Work out the finished part from the listing and answer in its coordinate system (mm). Face numbers are marked on the shaded views. A direction names the side the tool comes from. Coordinates: 2 decimals unless noted, no trailing zeros. Order: outer loops, then holes, each group sorted by start corner. A loop starts at its lowest first (then second) coordinate and runs counter-clockwise, first axis right, second up. Notation, with made-up numbers: M 4,-40 L 8,-40 A33 ccw 8,-3 Z; hole C -26.5,44 d2. An arc over 180 degrees is marked long. Use a Markdown table: item, result. Add a question column.
from build123d import *

# Parameters (mm, degrees)
SKETCH016_R           = 9.016071
PAD004_DEPTH          = 2
REVOLUTION003_ANGLE   = -140
POLARPATTERN001_COUNT = 2


with BuildPart() as part:
    # Sketch016 → Pad004 (new body)
    with BuildSketch(Plane.XY):
        Circle(SKETCH016_R)
    extrude(amount=-PAD004_DEPTH)

    # Sketch018 → Revolution003 (revolve)
    with BuildSketch(Plane.YZ):
        with BuildLine():
            Line((1.8, 0), (1.8, 8))
            Line((1.8, 8), (6.25, 8))
            ThreePointArc((6.25, 6), (6.5, 7), (6.25, 8))
            Line((6.25, 6), (6.25, 0))
            Line((6.25, 0), (1.8, 0))
        make_face()
    revolution003 = revolve(axis=Axis((0, 0, 0), (0, 0, 1)), revolution_arc=REVOLUTION003_ANGLE)

    # PolarPattern001: Revolution003 ×2 about axis
    polarpattern001_axis = Axis((0, 0, 0), (0, 0, 1))
    for i in range(1, POLARPATTERN001_COUNT):
        add(revolution003.rotate(polarpattern001_axis, i * 360 / POLARPATTERN001_COUNT))


solid = part.part
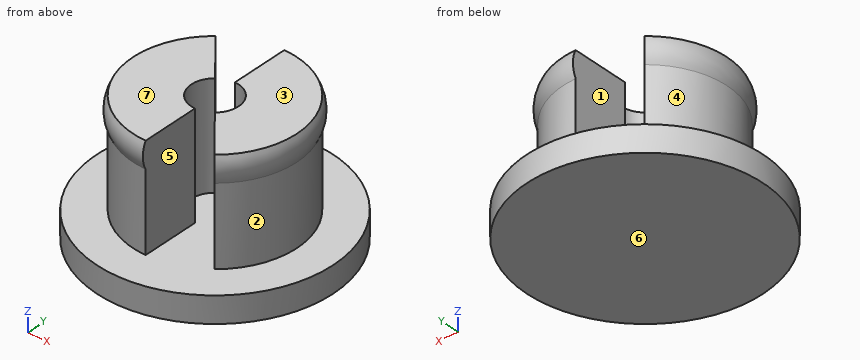
(1) Given P1, Ø1, axis at y = 5, z = 6, coming from the -X side; P2, Ø5, axis at x = 4, z = 4.5, coming from the -Y side; P3, Ø6, axis at x = 2.5, z = 6, coming from the +Y side, each flat-ended and moving along its own axis, determine where each tip first touches the part or whether it passes through.
(2) Which of the six approach directions +Z, -Z, +X, -X, +Y, -Y give full straight-line access (tool end or side, diameter ignored) to the marked faces 4, 5, 6 and 7?
(3) The mould has two halves that part along Z. Classify the marked faces 1, 2 and 3: pulls with the +Z half, pulls with the -Z half, needs draft (parallel to the pull), parting line crosses it, or undercut.
(4) Straight lines are drawn through the part: line 1 (Z direction, x = 1.5, y = -0.25); line 2 (X direction, y = 2.5, z = 2); line 3 (X direction, y = 0.25, z = 4) (3 decimals). For each, find the intervals that lie inside material, in ascending order.
(5) A cutting plane is placed at B-B on z = 1. Write down the section's boundary in (x, y), plus the area to 3 significant figures.
(6) A cutting plane is placed at C-C on x = 8. Write down the section's boundary in (y, z), plus the area to 3 significant figures.
(7) A cutting plane is placed at A-A on y = 0. Write down the section's boundary in (x, z) (3 decimals).
From the geometry:
| question | item | result |
|---|---|---|
| 1 | P1 | stops at x = -4.43 |
| 1 | P2 | stops at y = -4.98 |
| 1 | P3 | stops at y = 6.5 |
| 2 | face 4 | -X |
| 2 | face 5 | +Z, -Y |
| 2 | face 6 | -Z, +X, -X, +Y, -Y |
| 2 | face 7 | +Z, +X, -X, +Y, -Y |
| 3 | face 1 | needs draft |
| 3 | face 2 | undercut |
| 3 | face 3 | pulls with the +Z half |
| 4 | line 1 | z = -2 to 0 |
| 4 | line 2 | x = -5.73 to -2.1, 0 to 5.73 |
| 4 | line 3 | x = -6.245 to -1.783, 1.783 to 6.245 |
| 5 | outline | M -4.02,4.79 A6.25 ccw 0,-6.25 L 0,-1.8 A1.8 cw -1.16,1.38 Z; M 0,1.8 A1.8 cw 1.16,-1.38 L 4.02,-4.79 A6.25 ccw 0,6.25 Z |
| 5 | area | 87.5 mm2 |
| 6 | outline | M -4.16,-2 L 4.16,-2 L 4.16,0 L -4.16,0 Z |
| 6 | area | 16.6 mm2 |
| 7 | outline | M -9.016,-2 L 9.016,-2 L 9.016,0 L 6.25,0 L 6.25,6 A2.125 ccw 6.25,8 L 1.8,8 L 1.8,0 L -1.8,0 L -1.8,8 L -6.25,8 A2.125 ccw -6.25,6 L -6.25,0 L -9.016,0 Z |
